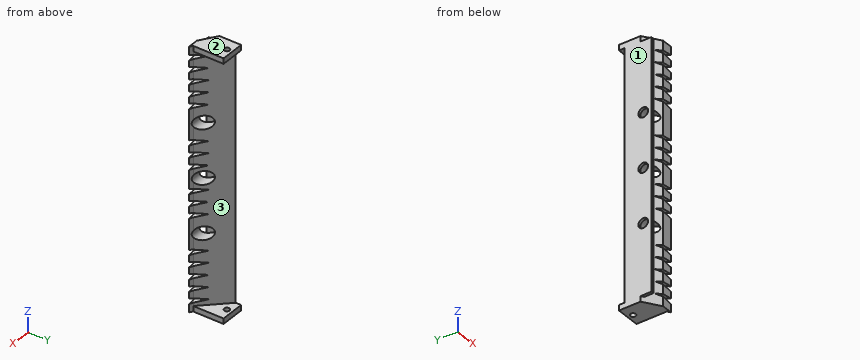
from build123d import *

# Parameters (mm, degrees)
BOSS_EXTRUDE1_DEPTH = 480
SKETCH2_R           = 5
BOSS_EXTRUDE2_DEPTH = 10
BOSS_EXTRUDE3_REACH = 482
CUT_EXTRUDE9_DEPTH  = 28
SKETCH14_W          = 460
SKETCH14_H          = 35
BOSS_EXTRUDE6_DEPTH = 5
SKETCH7_R           = 12.5
CUT_EXTRUDE8_DEPTH  = 56
SKETCH15_R          = 12.5
SKETCH15_R_2        = 9
BOSS_EXTRUDE7_DEPTH = 5


with BuildPart() as part:
    # Sketch1 → Boss-Extrude1 (new body)
    with BuildSketch(Plane.XY):
        Polygon((0, 0), (50, -35), (30, -35), (0, -15), align=None)
    extrude(amount=BOSS_EXTRUDE1_DEPTH)

    # Sketch2 → Boss-Extrude2 (add)
    with BuildSketch(Plane.XY.offset(480)):
        Polygon((0, -15), (0, 25), (44.349659334, 25), (44.349659334, -15), (44.349659334, -35), (30, -35), align=None)
        with Locations((22.174829667, 15)):
            Circle(SKETCH2_R, mode=Mode.SUBTRACT)
    boss_extrude2 = extrude(amount=-BOSS_EXTRUDE2_DEPTH)

    # Mirror1: Boss-Extrude2 across plane
    add(boss_extrude2.mirror(Plane.XY.offset(240)))

    # Sketch4 → Boss-Extrude3 (add, up to next)
    with BuildSketch(Plane.XY.offset(480), mode=Mode.PRIVATE) as boss_extrude3_sk1:
        Polygon((0, 0), (0, 15), (44.349659334, -31.044761534), align=None)
    boss_extrude3_tool1 = extrude(boss_extrude3_sk1.sketch, amount=-BOSS_EXTRUDE3_REACH, mode=Mode.PRIVATE) - part.part
    add(boss_extrude3_tool1.solids().sort_by_distance((14.78322, -5.348254, 480))[0])

    # Sketch3 → Cut-Extrude9 (cut, symmetric)
    with BuildSketch(Plane(origin=(0, 0, 0), x_dir=(0.819231921, -0.573462344, 0), z_dir=(0.573462344, 0.819231921, 0))):
        Polygon((61.032778079, -465), (31.032778079, -460), (61.032778079, -455), align=None)
        Polygon((61.032778079, -443), (31.032778079, -438), (61.032778079, -433), align=None)
        Polygon((61.032778079, -421), (31.032778079, -416), (61.032778079, -411), align=None)
        Polygon((61.032778079, -399), (31.032778079, -394), (61.032778079, -389), align=None)
        Polygon((61.032778079, -377), (31.032778079, -372), (61.032778079, -367), align=None)
        Polygon((61.032778079, -311), (31.032778079, -306), (61.032778079, -301), align=None)
        Polygon((61.032778079, -289), (31.032778079, -284), (61.032778079, -279), align=None)
        Polygon((61.032778079, -267), (31.032778079, -262), (61.032778079, -257), align=None)
        Polygon((61.032778079, -223), (31.032778079, -218), (61.032778079, -213), align=None)
        Polygon((61.032778079, -201), (31.032778079, -196), (61.032778079, -191), align=None)
        Polygon((61.032778079, -179), (31.032778079, -174), (61.032778079, -169), align=None)
        Polygon((61.032778079, -113), (31.032778079, -108), (61.032778079, -103), align=None)
        Polygon((61.032778079, -91), (31.032778079, -86), (61.032778079, -81), align=None)
        Polygon((61.032778079, -69), (31.032778079, -64), (61.032778079, -59), align=None)
        Polygon((61.032778079, -47), (31.032778079, -42), (61.032778079, -37), align=None)
        Polygon((61.032778079, -25), (31.032778079, -20), (61.032778079, -15), align=None)
    extrude(amount=CUT_EXTRUDE9_DEPTH, both=True, mode=Mode.SUBTRACT)

    # Sketch14 → Boss-Extrude6 (add)
    with BuildSketch(Plane.ZY):
        with Locations((240, -17.5)):
            Rectangle(SKETCH14_W, SKETCH14_H)
    extrude(amount=-BOSS_EXTRUDE6_DEPTH)

    # Sketch7 → Cut-Extrude8 (cut)
    with BuildSketch(Plane.ZY):
        with Locations((240, -20)):
            Circle(SKETCH7_R)
        with Locations((340, -20)):
            Circle(SKETCH7_R)
        with Locations((140, -20)):
            Circle(SKETCH7_R)
    extrude(amount=-CUT_EXTRUDE8_DEPTH, mode=Mode.SUBTRACT)

    # Sketch15 → Boss-Extrude7 (add)
    with BuildSketch(Plane.ZY):
        with Locations((340, -20)):
            Circle(SKETCH15_R)
        with Locations((340, -20)):
            Circle(SKETCH15_R_2, mode=Mode.SUBTRACT)
        with Locations((240, -20)):
            Circle(SKETCH15_R)
        with Locations((240, -20)):
            Circle(SKETCH15_R_2, mode=Mode.SUBTRACT)
        with Locations((140, -20)):
            Circle(SKETCH15_R)
        with Locations((140, -20)):
            Circle(SKETCH15_R_2, mode=Mode.SUBTRACT)
    extrude(amount=-BOSS_EXTRUDE7_DEPTH)


solid = part.part
Here's how the part is built. I have some questions about the finished solid (model axes, mm). Face numbers are marked on the shaded views. Round coordinates to 2 decimals unless told otherwise and drop trailing zeros. Order: outer loops, then holes, each group sorted by start corner. A loop starts at its lowest first (then second) coordinate and runs counter-clockwise, first axis right, second up. Notation, with made-up numbers: (24, 63) -> (41, 63) arc R5 cw to (41, 69) -> close; hole circle Ø9 at (56.5, 46). An arc over 180 degrees is marked (long way). Return JSON: item names as keys, results as strings.
Q1. If we mould it in two halves opening along Z, with no side actions, what happens to the marked faces 1, 2 and 3? For each: released by +Z, released by -Z, zero draft, split by the parting line, or undercut.
Filled sheet:
{"face 1": "zero draft", "face 2": "released by +Z", "face 3": "undercut"}
Q2. I need wall thicknesses on line 1 along Z through (x, y) = (17, -20); line 2 along Z through (x, y) = (32.5, 4.5); line 3 along Y through (x, z) = (32, 240). Which ranges of each line are inside material? Lowest first, please. Write a range as from..to.
Filled sheet:
{"line 1": "z = 0..127.5, 152.5..227.5, 252.5..327.5, 352.5..480", "line 2": "z = 0..10, 470..480", "line 3": "y = -35..-32.5"}
Q3. If we section it at A-A on z = 240: List the corners of the cut face in (x, y) for me, plus the area to 3 significant figures.
Filled sheet:
{"outline": "(0, -35) -> (5, -35) -> (5, -29) -> (0, -29) -> close; (0, -11) -> (5, -11) -> (5, -7.5) -> (21.67, -7.5) -> (0, 15) -> close; (26.25, -32.5) -> (30, -35) -> (50, -35) -> (46.43, -32.5) -> close", "area": "342 mm^2"}
Q4. If we section it at B-B on x = 40: Give the number of separate pieces and of enclosed holes in the cut face, plus the area to 3 significant figures.
Filled sheet:
{"separate pieces": "17", "enclosed holes": "0", "area": "3,950 mm^2"}
Q5. For pin 1 Ø12 at (x, z) = (26.5, 361.5) entering from -Y; pin 2 Ø14 at (y, z) = (-27, 240.5) entering from +X; pin 3 Ø3 at (x, z) = (26, 423.5) entering from +Y; pin 4 Ø20.5 at (y, z) = (-20, 340) entering from +X, each with a flat end and sliding along its axis, tell me the tip position at first contact or that it passes through.
Filled sheet:
{"pin 1": "stops at y = -35", "pin 2": "stops at x = 48.57", "pin 3": "stops at y = -10.44", "pin 4": "stops at x = 5"}
Q6. If we section it at C-C on z = 29.5: List the corners of the cut face in (x, y) for me, plus the area to 3 significant figures.
Filled sheet:
{"outline": "(0, -35) -> (5, -35) -> (5, -18.33) -> (30, -35) -> (50, -35) -> (44.35, -31.04) -> (0, 15) -> close", "area": "999 mm^2"}
